Geometry: final body of the model. Coordinates: model frame, mm. Round coordinates to 2 decimals unless told otherwise and drop trailing zeros. Loops run counter-clockwise (first coordinate to the right, second up) from the corner with the lowest first, then second, coordinate; pieces in that order, holes last. Notation, with made-up numbers: M -9.75,66 L 25.25,66 A26 cw 25.25,103 Z; hole C 46.25,-15.75 d6. An arc over 180 degrees is marked long. Answer as a JSON object with one key per item and string values.
from build123d import *

# Parameters (mm, degrees)
CROQUIS1_W              = 191.3
CROQUIS1_H              = 109
CROQUIS1_W_2            = 161.5
CROQUIS1_H_2            = 92
SALIENTE_EXTRUIR1_DEPTH = 9.2
CROQUIS2_W              = 175.3
CROQUIS2_H              = 101
CROQUIS2_W_2            = 161.5
CROQUIS2_H_2            = 92
CORTAR_EXTRUIR1_DEPTH   = 7.2
CROQUIS3_W              = 4
CROQUIS3_H              = 53
CORTAR_EXTRUIR2_DEPTH   = 3
REDONDEO3_R             = 2


with BuildPart() as part:
    # Croquis1 → Saliente-Extruir1 (new body)
    with BuildSketch(Plane(origin=(0, 0, 0), x_dir=(1, 0, 0), z_dir=(0, 1, 0))):
        with Locations((95.65, 54.5)):
            Rectangle(CROQUIS1_W, CROQUIS1_H)
        with Locations((95.65, 56.5)):
            Rectangle(CROQUIS1_W_2, CROQUIS1_H_2, mode=Mode.SUBTRACT)
    extrude(amount=SALIENTE_EXTRUIR1_DEPTH)

    # Croquis2 → Cortar-Extruir1 (cut)
    with BuildSketch(Plane.XZ):
        with Locations((95.65, -54.5)):
            Rectangle(CROQUIS2_W, CROQUIS2_H)
        with Locations((95.65, -56.5)):
            Rectangle(CROQUIS2_W_2, CROQUIS2_H_2, mode=Mode.SUBTRACT)
    extrude(amount=-CORTAR_EXTRUIR1_DEPTH, mode=Mode.SUBTRACT)

    # Croquis3 → Cortar-Extruir2 (cut)
    with BuildSketch(Plane.XZ):
        with Locations((4, -54.5)):
            Rectangle(CROQUIS3_W, CROQUIS3_H)
    extrude(amount=-CORTAR_EXTRUIR2_DEPTH, mode=Mode.SUBTRACT)

    # Redondeo3
    redondeo3_edges = [part.edges().sort_by_distance(p)[0] for p in [
        (0, 0, -54.5),
        (0, 4.6, -109),
        (95.65, 0, -109),
        (191.3, 4.6, -109),
        (191.3, 0, -54.5),
        (0, 4.6, 0),
        (191.3, 4.6, 0),
        (95.65, 0, 0),
        (14.9, 9.2, -56.5),
        (95.65, 9.2, -10.5),
        (176.4, 9.2, -56.5),
        (95.65, 9.2, -102.5),
        (95.65, 9.2, -109),
        (191.3, 9.2, -54.5),
        (95.65, 9.2, 0),
        (0, 9.2, -54.5),
    ]]
    fillet(redondeo3_edges, radius=REDONDEO3_R - 0.0001)  # a hair under: the kernel refuses the full size


solid = part.part
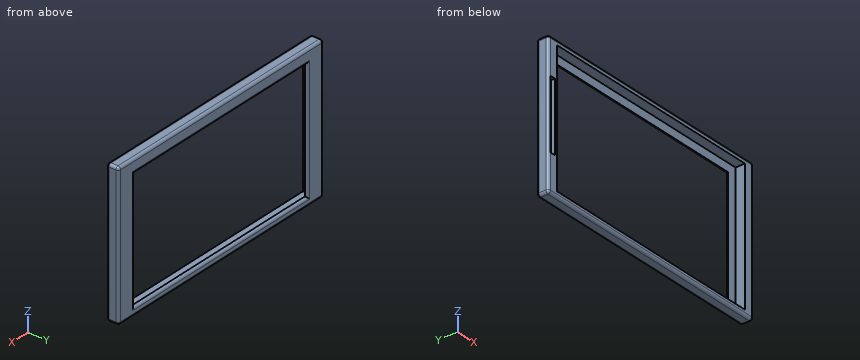
1) Pin query (flat end, axial travel): P1, Ø1.5, axis at y = 1, z = -49.5, coming from the +X side; P2, Ø2, axis at x = 4, z = -48.5, coming from the -Y side. Return the tip coordinate at first contact, or that it passes through.
Results:
{"P1": "x = 191.28", "P2": "y = 3"}
2) Section query C-C (y = 4.5). Return the cut outline in (x, z), and give its area (3 significant figures).
Results:
{"outline": "M 0,-107 A2 ccw 2,-109 L 189.3,-109 A2 ccw 191.3,-107 L 191.3,-2 A2 ccw 189.3,0 L 2,0 A2 ccw 0,-2 Z; hole M 8,-105 L 183.3,-105 L 183.3,-4 L 8,-4 Z", "area": "3,140 mm2"}
3) Ray query, line 1 (X direction, y = 2.75, z = -43.5); line 2 (Z direction, x = 85, y = 4.25); line 3 (X direction, y = 4.75, z = -66.5). Return the intervals inside material, ascending.
Results:
{"line 1": "0 to 2, 6 to 8, 183.3 to 191.3", "line 2": "-109 to -105, -4 to 0", "line 3": "0 to 8, 183.3 to 191.3"}
